Autodesk Inventor part; units mm, degrees
ref_plane "YZ Plane" through (0, 0, 0) normal (1, 0, 0) x (0, 1, 0)
ref_plane "XZ Plane" through (0, 0, 0) normal (0, 1, 0) x (-1, 0, 0)
ref_plane "XY Plane" through (0, 0, 0) normal (0, 0, 1) x (1, 0, 0)
sketch "Sketch1" plane through (0, 0, 0) normal (0, 1, 0) x (-1, 0, 0)
  line L0 (0, 0) -> (0, -61.8744)
  line L1 (0, 0) -> (-3.4036, 0)
  line L2 (0, -61.8744) -> (-3.4036, -61.8744)
  line L3 (-3.4036, 0) -> (-6.5786, -15.5321)
  line L4 (-6.5786, -15.5321) -> (-3.4036, -31.0642)
  line L5 (-3.4036, -31.0642) -> (-6.5786, -46.3423)
  line L6 (-6.5786, -46.3423) -> (-3.4036, -61.8744)
  dimension "d0" = 61.8744
  dimension "d1" = 3.4036
  dimension "d2" = 3.4036
  dimension "d3" = 15.5321
  dimension "d4" = 31.0642
  dimension "d5" = 15.5321
  dimension "d6" = 3.175
  dimension "d7" = 3.175
extrude "Extrusion1" add sketch "Sketch1" along normal blind 5.8166
sketch "Sketch2" plane through (0, 0, 0) normal (0, 0, 1) x (1, 0, 0)
  line L0 (3.4036, 0) -> (0, 0)
  line L1 (0, 5.8166) -> (1.651, 5.8166)
  line L2 (1.651, 5.8166) -> (1.651, 0)
  line L3 (1.651, 0) -> (0, 0)
  line L4 (0, 0) -> (0, 5.8166)
  dimension "d10" = 1.651
sketch "Sketch3" plane through (3.4036, 0, -61.8744) normal (0, 0, -1) x (-1, 0, 0)
  line L0 (0, 0) -> (3.4036, 0)
  line L1 (3.4036, 5.8166) -> (1.7526, 5.8166)
  line L2 (1.7526, 5.8166) -> (1.7526, 0)
  line L3 (1.7526, 0) -> (3.4036, 0)
  line L4 (3.4036, 0) -> (3.4036, 5.8166)
  dimension "d11" = 1.651
extrude "Extrusion2" add sketch "Sketch3" along normal blind 2.5654
extrude "Extrusion3" add sketch "Sketch2" along normal blind 2.5654
properties part number "Short_insert_CPY3_CPY"
Input: part model. Units: mm. Frame: model coordinates. A direction names the side the tool comes from. Round coordinates to 2 decimals unless told otherwise and drop trailing zeros. Loops run counter-clockwise (first coordinate to the right, second up) from the corner with the lowest first, then second, coordinate; pieces in that order, holes last. Notation, with made-up numbers: (-3, -24) -> (30, -24) arc R21 ccw to (30, -2) -> close; hole circle Ø8 at (-5.5, 87). An arc over 180 degrees is marked (long way). Use one line per item in the form item = value. Start each with the question number.
Item 1: Section query B-B on x = 5.75. Return the cut outline in (y, z).
Item 2: Contact query for flat-ended pins moving along their axis: pin 1 Ø1.4 at (x, y) = (3, 2.5) entering from -Z; pin 2 Ø2 at (y, z) = (4, 1.5) entering from +X; pin 3 Ø1.4 at (x, y) = (3, 2) entering from +Z. Output: stop coordinate, or through.
Item 3: Set-up query: faces 4 (the face through (1.651, 3, -63)), 5 (the face through (1.651, 3, 1)), 6 (the face through (3, 5.817, -31)), 7 (the face through (4.97, 2.87, -38.6)). Return all of +Z, -Z, +X, -X, +Y, -Y with unobstructed straight access to the full face (end or side cutting, diameter ignored); none if empty.
Item 4: Mould query, pull axis Z, two halves, no side actions, for faces 1 (the face through (4.97, 2.87, -7.66)), 2 (the face through (5.013, 2.868, -23.189)), 3 (the face through (1, 3, -64.44)). Classes: pulls with the +Z half, pulls with the -Z half, needs draft (parallel to the pull), parting line crosses it, or undercut.
Item 5: Section query A-A on y = 3.4. Return the cut outline in (x, z), then the cut area to 3 significant figures.
Item 6: Section query D-D on z = -20. Return the cut outline in (x, y), then the cut area to 3 significant figures.
Item 7: Section query C-C on x = 2.5. Return the cut outline in (y, z).
Item 8: Material intervals for L1, parallel to Z at x = 3, y = 0.4; L2, parallel to X at y = 3.65, z = -31; L3, parallel to X at y = 0.9, z = -37.5, sorted ascending. Write a range as from..to.
Ans:
q1.outline = (0, -50.4) -> (5.82, -50.4) -> (5.82, -42.36) -> (0, -42.36) -> close; (0, -19.59) -> (5.82, -19.59) -> (5.82, -11.48) -> (0, -11.48) -> close
q2.pin_1 = -61.87
q2.pin_2 = 1.65
q2.pin_3 = 0
q3.face_4 = -Z, +X, +Y, -Y
q3.face_5 = +Z, +X, +Y, -Y
q3.face_6 = +Z, -Z, +X, -X, +Y
q3.face_7 = +X, +Y, -Y
q4.face_1 = pulls with the +Z half
q4.face_2 = undercut
q4.face_3 = pulls with the -Z half
q5.outline = (0, -64.44) -> (1.65, -64.44) -> (1.65, -61.87) -> (3.4, -61.87) -> (6.58, -46.34) -> (3.4, -31.06) -> (6.58, -15.53) -> (3.4, 0) -> (1.65, 0) -> (1.65, 2.57) -> (0, 2.57) -> close
q5.area = 317 mm^2
q6.outline = (0, 0) -> (5.67, 0) -> (5.67, 5.82) -> (0, 5.82) -> close
q6.area = 33.0 mm^2
q7.outline = (0, -61.87) -> (5.82, -61.87) -> (5.82, 0) -> (0, 0) -> close
q8.L1 = -61.87..0
q8.L2 = 0..3.42
q8.L3 = 0..4.74
